Geometry check sheet. Reference: the model listing, model coordinates, mm. A direction names the side the tool comes from. Round coordinates to 2 decimals unless told otherwise and drop trailing zeros. Order: outer loops, then holes, each group sorted by start corner. A loop starts at its lowest first (then second) coordinate and runs counter-clockwise, first axis right, second up.
(1) Thickness scan on L1, parallel to Y at x = 0, z = 9.7; L2, parallel to Y at x = 0, z = 2.75; L3, parallel to Z at x = 3.5, y = 7.5. Record the ranges inside material, lowest first.
(2) Cross-section at C-C on z = 8.25. Enter the section's corners in (x, y).
(3) Draft check along X on faces 4 (the face through (-6, 0, 5)), 5 (the face through (-3.47, 15.62, 4.94)), 6 (the face through (0, 7, 0)). Enter one of: pulls with the +X half, pulls with the -X half, needs draft (parallel to the pull), parting line crosses it, or undercut.
(4) Gauge pin test, flat ends, axial feed: P1, Ø2, axis at y = -11.5, z = 5.5, coming from the -X side; P2, Ø1.5, axis at y = 4.5, z = 4, coming from the +X side; P3, Ø2, axis at x = -2.5, y = -9, coming from the -Z side. Record the tip position at first contact, or that the pin passes through.
(5) Set-up check for faces 1 (the face through (-12, -8, 0)), 2 (the face through (12.932, -5.362, 9.754)), 3 (the face through (1.73, -7.81, 0.25)): record each of +Z, -Z, +X, -X, +Y, -Y from which the full face is reachable in a straight line by a thin tool's end or side.
Autodesk Inventor part; units mm, degrees
ref_plane "YZ Plane" through (0, 0, 0) normal (1, 0, 0) x (0, 1, 0)
ref_plane "XZ Plane" through (0, 0, 0) normal (0, 1, 0) x (-1, 0, 0)
ref_plane "XY Plane" through (0, 0, 0) normal (0, 0, 1) x (1, 0, 0)
sketch "Sketch1" plane through (0, 0, 0) normal (0, 0, 1) x (1, 0, 0)
  circle A0 centre (0, 0) radius 6
  circle A1 centre (0, 0) radius 16
  dimension "d0" = 12
  dimension "d1" = 32
extrude "Extrusion1" add sketch "Sketch1" along normal blind 10
sketch "Sketch2" plane through (0, 0, 10) normal (0, 0, 1) x (1, 0, 0)
  circle A0 centre (0, 0) radius 6
  circle A1 centre (0, 0) radius 6
  circle A2 centre (0, 0) radius 16
  circle A3 centre (0, 0) radius 8
  circle A4 centre (0, 0) radius 14
  dimension "d4" = 2
  dimension "d5" = 2
extrude "Extrusion2" cut sketch "Sketch2" against normal blind 0.5 contours A4
sketch "Sketch3" plane through (0, 0, 0) normal (0, 0, -1) x (-1, 0, 0)
  circle A0 centre (0, 0) radius 8
  circle A1 centre (0, 0) radius 14
extrude "Extrusion3" cut sketch "Sketch3" against normal blind 0.5
chamfer "Chamfer1" distance 0.5 angle 45 4 edges at (-16, 0, 10) (-16, 0, 0) (-6, 0, 10) (-6, 0, 0)
properties part number "6201-2RS" material "Stainless Steel"
Found:
1. L1: y = -15.8 to -14, -8 to -6.2, 6.2 to 8, 14 to 15.8
1. L2: y = -16 to -6, 6 to 16
1. L3: z = 0.5 to 9.5
2. outline: circle Ø32 at (0, 0); hole circle Ø12 at (0, 0)
3. face 4: undercut
3. face 5: parting line crosses it
3. face 6: needs draft
4. P1: stops at x = -12.07
4. P2: stops at x = 15.55
4. P3: stops at z = 0.5
5. face 1: -Z, +X, -X, +Y, -Y
5. face 2: +Z
5. face 3: -Z
